```python
from build123d import *

# Parameters (mm, degrees)
EXTRUDE2_DEPTH      = 21.122535874
EXTRUDE2_DEPTH_BACK = 21.122535874
SKETCH3_W           = 7.52868736
SKETCH3_H           = 2
EXTRUDE3_DEPTH      = 21.122535963


with BuildPart() as part:
    # Sketch1 → Revolve1 (revolve)
    with BuildSketch(Plane(origin=(0, 0, 0), x_dir=(0, 0, -1), z_dir=(1, 0, 0)), mode=Mode.PRIVATE) as revolve1_sk:
        Polygon((0, 0), (0, 7.73110418), (-3.5, 9.005), (-15.109749167, 9.005), (-15.58, 7.25), (-15.58, 0), align=None)
    revolve(revolve1_sk.sketch.rotate(Axis((0, 0, 0), (0, 0, 1)), 90), axis=Axis((0, 0, 0), (0, 0, 1)))

    # Sketch2 → Extrude2 (cut, two sides: drawn at the far end of the back side and taken through both)
    with BuildSketch(Plane(origin=(0, 0, 0), x_dir=(0, -1, 0), z_dir=(1, 0, 0)).offset(-EXTRUDE2_DEPTH_BACK)):
        with BuildLine():
            Line((-0.152741588, -15.050887618), (-0.6, -15.58))
            Line((-0.6, -15.58), (0.6, -15.58))
            Line((0.6, -15.58), (0.152741588, -15.050887618))
            ThreePointArc((0.152741588, -15.050887618), (0, -14.98), (-0.152741588, -15.050887618))
        make_face()
    extrude(amount=EXTRUDE2_DEPTH + EXTRUDE2_DEPTH_BACK, mode=Mode.SUBTRACT)

    # Sketch3 → Extrude3 (cut, through all)
    with BuildSketch(Plane.XY.offset(15.58)):
        with Locations((0, 9.91)):
            Rectangle(SKETCH3_W, SKETCH3_H)
    extrude(amount=-EXTRUDE3_DEPTH, mode=Mode.SUBTRACT)


solid = part.part
```
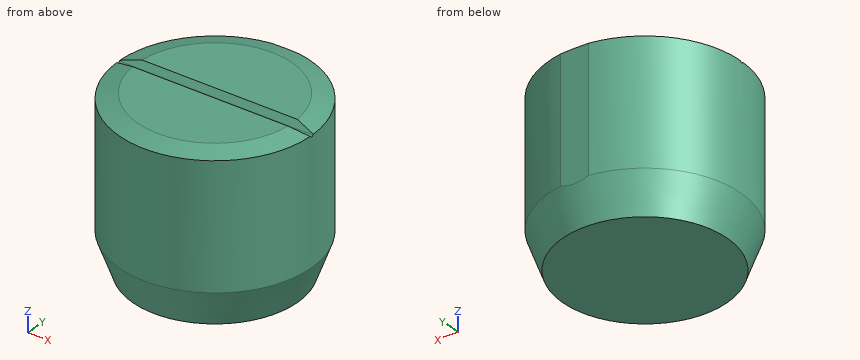
Can you work these out from the model? Positions are in its coordinate system, mm. Coordinates: 2 decimals unless noted, no trailing zeros. Order: outer loops, then holes, each group sorted by start corner. A loop starts at its lowest first (then second) coordinate and runs counter-clockwise, first axis right, second up. Notation, with made-up numbers: (31.25, 43.5) - (71.25, 43.5) arc R17 ccw to (71.25, 69.5) - close; hole circle Ø5 at (69, 9.5). An arc over 180 degrees is marked (long way). Answer in a Markdown table with one row per item.
1. Suppose I cut it at A-A (x = 0). Please give me the cut outline in (y, z) (3 decimals).
Reply:
| item | result |
|---|---|
| outline | (-9.005, 3.5) - (-7.731, 0) - (7.731, 0) - (8.91, 3.239) - (8.91, 15.135) - (7.25, 15.58) - (0.6, 15.58) - (0.153, 15.051) arc R0.2 cw to (-0.153, 15.051) - (-0.6, 15.58) - (-7.25, 15.58) - (-9.005, 15.11) - close |
2. For pin 1 (6 mm diameter, centred on y = -3.5, z = 3.5, fed in from -X); pin 2 (1.5 mm diameter, centred on y = 6.5, z = 13, fed in from +X), each with a flat end and sliding along its axis, tell me the tip position at first contact or that it passes through.
Reply:
| item | result |
|---|---|
| pin 1 | stops at x = -8.99 |
| pin 2 | stops at x = 6.93 |
3. If I drill on line 1 along X through (y, z) = (-2.25, 14); line 2 along Y through (x, z) = (-4.75, 6.25); line 3 along Z through (x, y) = (-3.25, 6.75), over which ranges is the centre line in solid material (lowest first)?
Reply:
| item | result |
|---|---|
| line 1 | x = -8.72 to 8.72 |
| line 2 | y = -7.65 to 7.65 |
| line 3 | z = 0 to 15.52 |
4. Suppose I cut it at B-B (z = 6.25). Please give me the cut outline in (x, y) (3 decimals), and give its area (3 significant figures).
Reply:
| item | result |
|---|---|
| outline | (-1.305, 8.91) arc R9.005 ccw (long way) to (1.305, 8.91) - close |
| area | 255 mm^2 |
